from build123d import *

# Parameters (mm, degrees)
SKETCH1_W                      = 127
SKETCH1_H                      = 60
BOSS_EXTRUDE1_DEPTH            = 10
CUT_EXTRUDE1_START             = -5.08
SKETCH3_R                      = 7.525
CUT_EXTRUDE1_DEPTH             = 24.05
CUT_EXTRUDE2_REACH             = 127.954
SKETCH4_R                      = 4.25
CUT_EXTRUDE2_DIRECTION_2_REACH = 127.954
CUT_EXTRUDE3_START             = -68.74
SKETCH5_R                      = 5.25
SKETCH5_R_2                    = 4.25
CUT_EXTRUDE3_DEPTH             = 68.74
SKETCH6_W                      = 15.875
SKETCH6_H                      = 10
CUT_EXTRUDE4_DEPTH             = 19.05
M3_CLEARANCE_HOLE1_D           = 3.4
CUT_EXTRUDE5_START             = -6.35
CUT_EXTRUDE5_DEPTH             = 5
M3X0_5_TAPPED_HOLE1_D          = 2.5
SKETCH12_W                     = 7.62
SKETCH12_H                     = 8.4125
CUT_EXTRUDE6_DEPTH             = 113.48645474
CUT_EXTRUDE7_REACH             = 72.938
SKETCH13_R                     = 12.7


with BuildPart() as part:
    # Sketch1 → Boss-Extrude1 (new body)
    with BuildSketch(Plane(origin=(0, 0, 0), x_dir=(1, 0, 0), z_dir=(0, 1, 0))):
        Rectangle(SKETCH1_W, SKETCH1_H)
    extrude(amount=BOSS_EXTRUDE1_DEPTH)

    # Sketch3 → Cut-Extrude1 (cut)
    with BuildSketch(Plane.ZY.offset(63.5).offset(CUT_EXTRUDE1_START)):
        with Locations((-20, 10)):
            Circle(SKETCH3_R)
        with Locations((20, 10)):
            Circle(SKETCH3_R)
    cut_extrude1 = extrude(amount=-CUT_EXTRUDE1_DEPTH, mode=Mode.SUBTRACT)

    # Mirror1: Cut-Extrude1 across plane
    add(cut_extrude1.mirror(Plane(origin=(0, 0, 0), x_dir=(0, 0, 1), z_dir=(1, 0, 0))), mode=Mode.SUBTRACT)

    # Sketch4 → Cut-Extrude2 (cut, up to next)
    with BuildSketch(Plane(origin=(-58.42, 0, 0), x_dir=(0, 0, -1), z_dir=(1, 0, 0)), mode=Mode.PRIVATE) as cut_extrude2_sk1:
        with Locations((20, 10)):
            Circle(SKETCH4_R)
    cut_extrude2_tool1 = extrude(cut_extrude2_sk1.sketch, amount=-CUT_EXTRUDE2_REACH, mode=Mode.PRIVATE) & part.part
    cut_extrude2 = cut_extrude2_tool1.solids().sort_by_distance((-58.42, 10, -20))[0]
    add(cut_extrude2, mode=Mode.SUBTRACT)

    # Cut-Extrude2 direction 2: up to this face of the body (flat: up to its plane)
    cut_extrude2_direction_2_end = Plane(part.part.faces().sort_by_distance((63.5, 5, 0))[0])
    # Sketch4 → Cut-Extrude2 direction 2 (cut, up to the picked face)
    with BuildSketch(Plane(origin=(-58.42, 0, 0), x_dir=(0, 0, -1), z_dir=(1, 0, 0)), mode=Mode.PRIVATE) as cut_extrude2_direction_2_sk1:
        with Locations((20, 10)):
            Circle(SKETCH4_R)
    cut_extrude2_direction_2_tool1 = split(extrude(cut_extrude2_direction_2_sk1.sketch, amount=CUT_EXTRUDE2_DIRECTION_2_REACH, mode=Mode.PRIVATE), bisect_by=cut_extrude2_direction_2_end, keep=Keep.BOTH, mode=Mode.PRIVATE)
    cut_extrude2_direction_2 = cut_extrude2_direction_2_tool1.solids().sort_by(Axis((-58.42, 10, -20), (1, 0, 0)))[0]
    add(cut_extrude2_direction_2, mode=Mode.SUBTRACT)

    # Mirror2: Cut-Extrude2, Cut-Extrude2 direction 2 across plane
    add(cut_extrude2.mirror(Plane.XY), mode=Mode.SUBTRACT)
    add(cut_extrude2_direction_2.mirror(Plane.XY), mode=Mode.SUBTRACT)

    # Sketch5 → Cut-Extrude3 (cut)
    with BuildSketch(Plane(origin=(34.37, 0, 0), x_dir=(0, 0, -1), z_dir=(1, 0, 0)).offset(CUT_EXTRUDE3_START)):
        with Locations((-20, 10)):
            Circle(SKETCH5_R)
        with Locations((-20, 10)):
            Circle(SKETCH5_R_2, mode=Mode.SUBTRACT)
    cut_extrude3 = extrude(amount=CUT_EXTRUDE3_DEPTH, mode=Mode.SUBTRACT)

    # Mirror3: Cut-Extrude3 across plane
    add(cut_extrude3.mirror(Plane.XY), mode=Mode.SUBTRACT)

    # Sketch6 → Cut-Extrude4 (cut)
    with BuildSketch(Plane.ZY.offset(63.5)):
        with Locations((0, 5)):
            Rectangle(SKETCH6_W, SKETCH6_H)
    cut_extrude4 = extrude(amount=-CUT_EXTRUDE4_DEPTH, mode=Mode.SUBTRACT)

    # Mirror4: Cut-Extrude4 across plane
    add(cut_extrude4.mirror(Plane(origin=(0, 0, 0), x_dir=(0, 0, 1), z_dir=(1, 0, 0))), mode=Mode.SUBTRACT)

    # M3 Clearance Hole1 (through all)
    with Locations(Plane.ZY.offset(44.45)):
        with Locations((-3.5375, 4.4)):
            Hole(M3_CLEARANCE_HOLE1_D / 2)

    # Sketch9 → Cut-Extrude5 (cut)
    with BuildSketch(Plane.ZY.offset(44.45).offset(CUT_EXTRUDE5_START)):
        Polygon((-0.7875, 0), (-0.7875, 5.98771324), (-3.5375, 7.575426481), (-6.2875, 5.98771324), (-6.2875, 0), align=None)
    cut_extrude5 = extrude(amount=-CUT_EXTRUDE5_DEPTH, mode=Mode.SUBTRACT)

    # Mirror5: Cut-Extrude5 across plane
    add(cut_extrude5.mirror(Plane(origin=(0, 0, 0), x_dir=(0, 0, 1), z_dir=(1, 0, 0))), mode=Mode.SUBTRACT)

    # M3x0.5 Tapped Hole1 (through all)
    with Locations(Plane(origin=(0, 10, 0), x_dir=(1, 0, 0), z_dir=(0, 1, 0))):
        with Locations((-31.75, -11.1125), (31.75, -11.1125), (-31.75, 11.1125), (31.75, 11.1125), (0, -11.1125), (0, 11.1125)):
            Hole(M3X0_5_TAPPED_HOLE1_D / 2)

    # Sketch12 → Cut-Extrude6 (cut, through all)
    with BuildSketch(Plane.ZY.offset(44.45)):
        with Locations((4.1275, 4.20625)):
            Rectangle(SKETCH12_W, SKETCH12_H)
    extrude(amount=-CUT_EXTRUDE6_DEPTH, mode=Mode.SUBTRACT)

    # Sketch13 → Cut-Extrude7 (cut, up to next)
    with BuildSketch(Plane.XZ, mode=Mode.PRIVATE) as cut_extrude7_sk1:
        with Locations((5.1218, 40.16)):
            Circle(SKETCH13_R)
    cut_extrude7_tool1 = extrude(cut_extrude7_sk1.sketch, amount=-CUT_EXTRUDE7_REACH, mode=Mode.PRIVATE) & part.part
    # Sketch13 → Cut-Extrude7 (cut, up to next)
    with BuildSketch(Plane.XZ, mode=Mode.PRIVATE) as cut_extrude7_sk2:
        with Locations((47.4218, 40.16)):
            Circle(SKETCH13_R)
    cut_extrude7_tool2 = extrude(cut_extrude7_sk2.sketch, amount=-CUT_EXTRUDE7_REACH, mode=Mode.PRIVATE) & part.part
    add(cut_extrude7_tool1.solids().sort_by_distance((5.1218, 0, 40.16))[0], mode=Mode.SUBTRACT)
    add(cut_extrude7_tool2.solids().sort_by_distance((47.4218, 0, 40.16))[0], mode=Mode.SUBTRACT)


solid = part.part
For this review, take the finished solid that the model builds, in its own axes (mm). A direction names the side the tool comes from. Round coordinates to 2 decimals unless told otherwise and drop trailing zeros. Loops run counter-clockwise (first coordinate to the right, second up) from the corner with the lowest first, then second, coordinate; pieces in that order, holes last. Notation, with made-up numbers: (-4.75, -22) - (52.25, -22) arc R10 cw to (52.25, -14) - close; hole circle Ø3 at (78.25, -5.5). An arc over 180 degrees is marked (long way). Put each result on its own line as item: value. Start each with the question number.
1. Consider section A-A on x = -31.75. State the section outline as (y, z) points, plus the area to 3 significant figures.
2. Mouldability with a two-part tool opening along X and no side actions: class faces 6 (the cylindrical face through (30.595, 4.93, -10.634)), 7 (the flat face through (-63.5, 5, -19)), 8 (the flat face through (59, 5, 30)), 9 (the cylindrical face through (47.31, 4.93, 27.46)) as +X half, -X half, draft (parallel to the pull), parting line (faces both ways), or undercut.
3. Insertion check: P1, Ø3, axis at x = -16, z = 2.5, coming from the -Y side; P2, Ø2, axis at x = 31.75, z = -11.11, coming from the -Y side; P3, Ø5, axis at y = 4.5, z = -2, coming from the -X side; P4, Ø4.5, axis at y = 4.5, z = -4.5, coming from the +X side. Each pin has a flat end and moves straight along its axis. Give the tip position at first contact, or say it passes through.
4. Consider section C-C on x = 0. State the section outline as (y, z) points, plus the area to 3 significant figures.
5. Consider section B-B on z = 20. State the section outline as (x, y) points (3 decimals), plus the area to 3 significant figures.
6. For faces 1 (the flat face through (-1, 4, 0.318)), 2 (the flat face through (54, 5, -7.938)), 3 (the flat face through (-54, 5, -7.938)), 4 (the flat face through (-58.42, 5, 20)), 5 (the flat face through (36, 3, -0.788)), list the 3-axis set-ups (+Z, -Z, +X, -X, +Y, -Y) from which the entire face can be reached by the end or side of a thin tool; tool diameter is ignored.
7. For probe 1 along X at (y, z) = (4.25, -5.5); probe 2 along X at (y, z) = (8.75, 14); probe 3 along Z at (x, y) = (-31.75, 3.5), list the stretches that pass through material, from the lowest coordinate up. Write a range as [from, to].
Result sheet:
1. outline: (0, -30) - (10, -30) - (10, -25.25) arc R5.25 cw to (10, -14.75) - (10, -12.36) - (0, -12.36) - close; (0, -9.86) - (10, -9.86) - (10, 9.86) - (0, 9.86) - (0, 7.94) - (8.41, 7.94) - (8.41, 0.32) - (0, 0.32) - close; (0, 12.36) - (10, 12.36) - (10, 14.75) arc R5.25 cw to (10, 25.25) - (10, 30) - (0, 30) - close; hole circle Ø3.4 at (4.4, -3.54)
1. area: 390 mm^2
2. face 6: undercut
2. face 7: -X half
2. face 8: draft
2. face 9: undercut
3. P1: y = 8.41
3. P2: through
3. P3: x = -44.45
3. P4: x = 44.45
4. outline: (0, -30) - (10, -30) - (10, -25.25) arc R5.25 cw to (10, -14.75) - (10, -12.36) - (0, -12.36) - close; (0, -9.86) - (10, -9.86) - (10, 9.86) - (0, 9.86) - (0, 7.94) - (8.41, 7.94) - (8.41, 0.32) - (0, 0.32) - close; (0, 12.36) - (10, 12.36) - (10, 14.75) arc R5.25 cw to (10, 25.25) - (10, 28.54) - (0, 28.54) - close; hole circle Ø3.4 at (4.4, -3.54)
4. area: 376 mm^2
5. outline: (-63.5, 0) - (63.5, 0) - (63.5, 5.75) - (58.42, 5.75) - (58.42, 2.475) - (34.37, 2.475) - (34.37, 4.75) - (-34.37, 4.75) - (-34.37, 2.475) - (-58.42, 2.475) - (-58.42, 5.75) - (-63.5, 5.75) - close
5. area: 504 mm^2
6. face 1: +X, -X, -Y
6. face 2: +X, +Y, -Y
6. face 3: -X, +Y, -Y
6. face 4: +Y
6. face 5: -Y
7. probe 1: [-44.45, -38.1], [-33.1, 33.1], [38.1, 44.45]
7. probe 2: [-63.5, -58.42], [-34.37, 34.37], [58.42, 63.5]
7. probe 3: [-30, -12.36], [-9.86, -4.98], [-2.1, 0.32], [7.94, 9.86], [12.36, 30]
